from build123d import *

# Parameters (mm, degrees)
SKETCH1_W           = 70
SKETCH1_H           = 96
SKETCH1_R           = 1.6
BOSS_EXTRUDE1_DEPTH = 10
SKETCH2_R           = 1.25
CUT_EXTRUDE1_DEPTH  = 10


with BuildPart() as part:
    # Sketch1 → Boss-Extrude1 (new body)
    with BuildSketch(Plane.XZ.offset(-316.566699204)):
        with Locations((0, 23.58434623)):
            Rectangle(SKETCH1_W, SKETCH1_H)
        with Locations(Location((-27, 59.58434623, 0), (0, 0, 270))):
            Circle(SKETCH1_R, mode=Mode.SUBTRACT)
        with Locations(Location((27, 59.58434623, 0), (0, 0, 270))):
            Circle(SKETCH1_R, mode=Mode.SUBTRACT)
        with Locations(Location((-27, -12.41565377, 0), (0, 0, 270))):
            Circle(SKETCH1_R, mode=Mode.SUBTRACT)
        with Locations(Location((27, -12.41565377, 0), (0, 0, 270))):
            Circle(SKETCH1_R, mode=Mode.SUBTRACT)
    extrude(amount=BOSS_EXTRUDE1_DEPTH)

    # Sketch2 → Cut-Extrude1 (cut)
    with BuildSketch(Plane.ZY.offset(35)):
        with Locations((-20.41565377, 311.566699204)):
            Circle(SKETCH2_R)
        with Locations((67.58434623, 311.566699204)):
            Circle(SKETCH2_R)
    cut_extrude1 = extrude(amount=-CUT_EXTRUDE1_DEPTH, mode=Mode.SUBTRACT)

    # Mirror1: Cut-Extrude1 across plane
    add(cut_extrude1.mirror(Plane(origin=(0, 0, 0), x_dir=(0, 0, 1), z_dir=(1, 0, 0))), mode=Mode.SUBTRACT)


solid = part.part
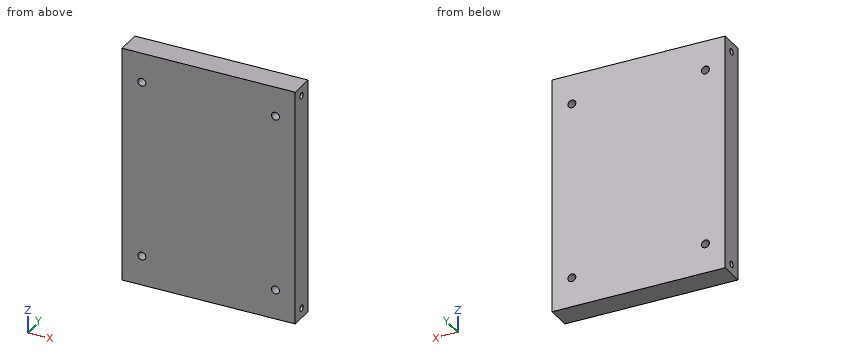
Build history of the part. All positions in model axes, mm. Coordinates: 2 decimals unless noted, no trailing zeros. Write each loop counter-clockwise with the first axis right and the second up, starting at its lowest first coordinate (ties: lowest second). Pieces come first, ordered by that corner, then holes. Notation, with made-up numbers: (-40, -13) -> (13, -13) arc R32 ccw to (13, 15) -> close; hole circle Ø6 at (48, -34). An arc over 180 degrees is marked (long way). Use CSV: the item, a comma, the result in double quotes. Start each with the question number.
Q1. Cut at B-B, the plane x = 27. List the corners of the cut face in (y, z).
Q2. Flat gauge pins, fed straight in: pin 1 Ø3 at (x, z) = (27, 59.58) entering from -Y; pin 2 Ø1.2 at (y, z) = (311.5, -20) entering from +X; pin 3 Ø1.5 at (y, z) = (311.57, 67.58) entering from -X. Where does each tip first touch, or does it go through?
Q3. Cut at A-A, the plane z = 59. List the corners of the cut face in (x, y).
Checked values:
1,outline,"(306.57, -24.42) -> (316.57, -24.42) -> (316.57, -14.02) -> (306.57, -14.02) -> close; (306.57, -10.82) -> (316.57, -10.82) -> (316.57, 57.98) -> (306.57, 57.98) -> close; (306.57, 61.18) -> (316.57, 61.18) -> (316.57, 71.58) -> (306.57, 71.58) -> close; hole circle Ø2.5 at (311.57, -20.42); hole circle Ø2.5 at (311.57, 67.58)"
2,pin 1,"passes through"
2,pin 2,"stops at x = 25"
2,pin 3,"stops at x = -25"
3,outline,"(-35, 306.57) -> (-28.49, 306.57) -> (-28.49, 316.57) -> (-35, 316.57) -> close; (-25.51, 306.57) -> (25.51, 306.57) -> (25.51, 316.57) -> (-25.51, 316.57) -> close; (28.49, 306.57) -> (35, 306.57) -> (35, 316.57) -> (28.49, 316.57) -> close"
